Geometry check sheet. Reference: the model listing, model coordinates, mm. Face numbers are marked on the shaded views. A direction names the side the tool comes from. Coordinates: 2 decimals unless noted, no trailing zeros. Write each loop counter-clockwise with the first axis right and the second up, starting at its lowest first coordinate (ties: lowest second). Pieces come first, ordered by that corner, then holes. Notation, with made-up numbers: (32, 86) -> (76, 86) arc R22 ccw to (76, 109) -> close; hole circle Ø8 at (-18, 25). An arc over 180 degrees is marked (long way). Answer in a Markdown table with one row per item. Add a question column.
1. Cross-section at A-A on z = 9.25. Record the cut outline in (x, y), and give its area (3 significant figures).
2. Scan lines: L1, parallel to Y at x = 24, z = 3.5; L2, parallel to Z at x = 23, y = -6; L3, parallel to Z at x = -28, y = -147. Record each from-to range of solid material in increasing order. Write a range as from..to.
3. Cross-section at D-D on x = 22.5. Record the cut outline in (y, z), and give its area (3 significant figures).
4. Mould release check, pull along Y, two halves, no side actions. Record for the marked faces 1 and 2: pulls with the +Y half, pulls with the -Y half, needs draft (parallel to the pull), parting line crosses it, or undercut.
5. Set-up check for the marked faces 3 and 4: record each of +Z, -Z, +X, -X, +Y, -Y from which the full face is reachable in a straight line by a thin tool's end or side.
6. Depth check by flat-ended pin: P1, Ø2, axis at y = -13.5, z = 4, coming from the +X side; P2, Ø2.5, axis at y = -98, z = 1, coming from the -X side; P3, Ø1.5, axis at x = 44.5, z = 1.5, coming from the +Y side. Enter the tip coordinate at first touch or a pass-through.
7. Cross-section at B-B on x = -3. Record the cut outline in (y, z).
8. Cross-section at C-C on y = -40. Record the cut outline in (x, z).
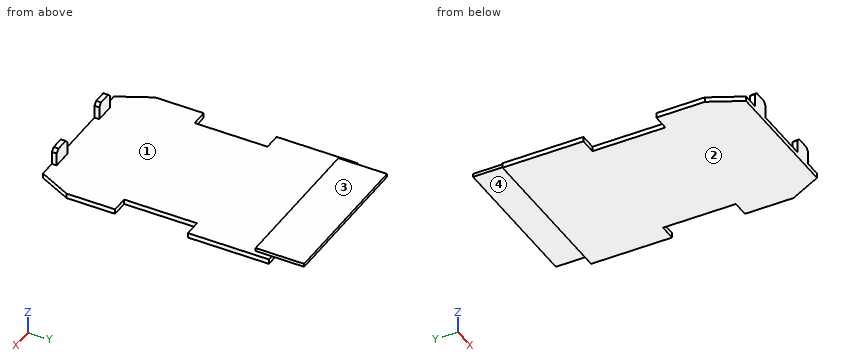
```python
from build123d import *

# Parameters (mm, degrees)
F1_DEPTH = 3
F2_W     = 12
F2_H     = 3
F3_DEPTH = 10
F4_SIZE  = 2
F5_W     = 93.5
F5_H     = 30
F6_DEPTH = 2


# Not quite as in the source:
# - a feature names something its author has since deleted; it is built from what else it names


with BuildPart() as f1:
    # F0 (on Top) → F1 (new body)
    with BuildSketch(Plane.XY):
        Polygon((50, -18.8796229661), (-50, -18.8796229661), (-50, -68.8796229661), (-39.780523628, -68.8796229661), (-39.780523628, -113.8796229661), (-50, -113.8796229661), (-50, -143.8796229661), (-40, -163.8796229661), (40, -163.8796229661), (50, -143.8796229661), (50, -113.8796229661), (39.780523628, -113.8796229661), (39.780523628, -68.8796229661), (50, -68.8796229661), align=None)
    extrude(amount=F1_DEPTH)

    # F2 (on face) → F3 (join)
    with BuildSketch(Plane.XY.offset(3)):
        with Locations((-24, -162.3796229661)):
            Rectangle(F2_W, F2_H)
        with Locations((24, -162.3796229661)):
            Rectangle(F2_W, F2_H)
    extrude(amount=F3_DEPTH)

    # F4
    f4_edges = [f1.edges().sort_by_distance(p)[0] for p in [
        (-18, -162.379623, 13),
        (-30, -162.379623, 13),
        (30, -162.379623, 13),
        (18, -162.379623, 13),
    ]]
    chamfer(f4_edges, length=F4_SIZE)

    # F5 (on face) → F6 (join)
    with BuildSketch(Plane.XY.offset(3)):
        with Locations((0, -13.8796229661)):
            Rectangle(F5_W, F5_H)
    extrude(amount=F6_DEPTH)


solid = f1.part
```
Results found:
| question | item | result |
|---|---|---|
| 1 | outline | (-30, -163.88) -> (-18, -163.88) -> (-18, -160.88) -> (-30, -160.88) -> close; (18, -163.88) -> (30, -163.88) -> (30, -160.88) -> (18, -160.88) -> close |
| 1 | area | 72.0 mm^2 |
| 2 | L1 | y = -163.88..-160.88, -28.88..1.12 |
| 2 | L2 | z = 3..5 |
| 2 | L3 | z = 0..3 |
| 3 | outline | (-163.88, 0) -> (-18.88, 0) -> (-18.88, 3) -> (1.12, 3) -> (1.12, 5) -> (-28.88, 5) -> (-28.88, 3) -> (-160.88, 3) -> (-160.88, 13) -> (-163.88, 13) -> close |
| 3 | area | 525 mm^2 |
| 4 | face 1 | undercut |
| 4 | face 2 | needs draft |
| 5 | face 3 | +Z, +X, -X, +Y |
| 5 | face 4 | -Z, +X, -X, +Y |
| 6 | P1 | stops at x = 46.75 |
| 6 | P2 | stops at x = -39.78 |
| 6 | P3 | stops at y = -18.88 |
| 7 | outline | (-163.88, 0) -> (-18.88, 0) -> (-18.88, 3) -> (1.12, 3) -> (1.12, 5) -> (-28.88, 5) -> (-28.88, 3) -> (-163.88, 3) -> close |
| 8 | outline | (-50, 0) -> (50, 0) -> (50, 3) -> (-50, 3) -> close |
